Build history of the part. All positions in model axes, mm. A direction names the side the tool comes from. Round coordinates to 2 decimals unless told otherwise and drop trailing zeros. Loops run counter-clockwise (first coordinate to the right, second up) from the corner with the lowest first, then second, coordinate; pieces in that order, holes last. Notation, with made-up numbers: (-7, 70.5) - (40, 70.5) arc R13 cw to (40, 89.5) - close; hole circle Ø9 at (-3, -39). An arc over 180 degrees is marked (long way). Put each result on its own line as item: value. Start each with the question number.
from build123d import *

# Parameters (mm, degrees)
ESQUISSE1_R             = 12.5
BOSS_EXTRU_1_DEPTH      = 54.5
ESQUISSE2_R             = 4
BOSS_EXTRU_2_DEPTH      = 1.35
ESQUISSE3_R             = 1.5
BOSS_EXTRU_3_DEPTH      = 15.7
ESQUISSE4_R             = 13
BOSS_EXTRU_4_DEPTH      = 32.9
ESQUISSE5_R             = 7.5
BOSS_EXTRU_5_DEPTH      = 2
ESQUISSE7_R             = 3
BOSS_EXTRU_6_DEPTH      = 20.8
ESQUISSE8_W             = 9.608231015
ESQUISSE8_H             = 12.440367957
ENL_V_MAT_EXTRU_1_DEPTH = 12
ESQUISSE9_R             = 1.5
ENL_V_MAT_EXTRU_2_DEPTH = 12
ESQUISSE10_R            = 13.05
BOSS_EXTRU_7_DEPTH      = 27
ESQUISSE11_R            = 12.55
BOSS_EXTRU_8_DEPTH      = 3
ESQUISSE12_R            = 1
ENL_V_MAT_EXTRU_4_DEPTH = 1


with BuildPart() as part:
    # Esquisse1 → Boss.-Extru.1 (new body)
    with BuildSketch(Plane.XY):
        Circle(ESQUISSE1_R)
    extrude(amount=BOSS_EXTRU_1_DEPTH)

    # Esquisse2 → Boss.-Extru.2 (add)
    with BuildSketch(Plane(origin=(0, 0, 0), x_dir=(-1, 0, 0), z_dir=(0, 0, -1))):
        with Locations(Location((0, 0, 0), (0, 0, 180))):
            Circle(ESQUISSE2_R)
    extrude(amount=BOSS_EXTRU_2_DEPTH)

    # Esquisse3 → Boss.-Extru.3 (add)
    with BuildSketch(Plane(origin=(0, 0, 0), x_dir=(-1, 0, 0), z_dir=(0, 0, -1))):
        Circle(ESQUISSE3_R)
    extrude(amount=BOSS_EXTRU_3_DEPTH)

    # Esquisse4 → Boss.-Extru.4 (add)
    with BuildSketch(Plane.XY.offset(54.5)):
        Circle(ESQUISSE4_R)
    extrude(amount=BOSS_EXTRU_4_DEPTH)

    # Esquisse5 → Boss.-Extru.5 (add)
    with BuildSketch(Plane.XY.offset(87.4)):
        Circle(ESQUISSE5_R)
    extrude(amount=BOSS_EXTRU_5_DEPTH)

    # Esquisse7 → Boss.-Extru.6 (add)
    with BuildSketch(Plane.XY.offset(87.4)):
        Circle(ESQUISSE7_R)
    extrude(amount=BOSS_EXTRU_6_DEPTH)

    # Esquisse8 → Enlèv. mat.-Extru.1 (cut)
    with BuildSketch(Plane.XY.offset(108.2)):
        with Locations((-0.725995737, 8.720183978)):
            Rectangle(ESQUISSE8_W, ESQUISSE8_H)
    extrude(amount=-ENL_V_MAT_EXTRU_1_DEPTH, mode=Mode.SUBTRACT)

    # Esquisse9 → Enlèv. mat.-Extru.2 (cut)
    with BuildSketch(Plane.XY.offset(87.4)):
        with Locations((-9.999727195, 0)):
            Circle(ESQUISSE9_R)
        with Locations((9.999727195, 0)):
            Circle(ESQUISSE9_R)
        with Locations((0, -10.073864879)):
            Circle(ESQUISSE9_R)
        with Locations((0, 9.926135121)):
            Circle(ESQUISSE9_R)
    extrude(amount=-ENL_V_MAT_EXTRU_2_DEPTH, mode=Mode.SUBTRACT)

    # Esquisse10 → Boss.-Extru.7 (add)
    with BuildSketch(Plane(origin=(0, 0, 54.5), x_dir=(-1, 0, 0), z_dir=(0, 0, -1))):
        Circle(ESQUISSE10_R)
    extrude(amount=-BOSS_EXTRU_7_DEPTH)

    # Esquisse11 → Boss.-Extru.8 (add)
    with BuildSketch(Plane(origin=(0, 0, 0), x_dir=(-1, 0, 0), z_dir=(0, 0, -1))):
        Circle(ESQUISSE11_R)
    extrude(amount=-BOSS_EXTRU_8_DEPTH)

    # Esquisse12 → Enlèv. mat.-Extru.4 (cut)
    with BuildSketch(Plane(origin=(0, 0, 0), x_dir=(-1, 0, 0), z_dir=(0, 0, -1))):
        with Locations((0, 8.5)):
            Circle(ESQUISSE12_R)
        with Locations((7.361215932, -4.25)):
            Circle(ESQUISSE12_R)
        with Locations((0, -8.5)):
            Circle(ESQUISSE12_R)
        with Locations((-7.361215932, -4.25)):
            Circle(ESQUISSE12_R)
        with BuildLine():
            Line((12.364465213, 2.15), (10.005928826, 2.15))
            Line((10.005928826, 2.15), (10.005928826, -0.65))
            Line((10.005928826, -0.65), (12.533156027, -0.65))
            ThreePointArc((12.533156027, -0.65), (12.527285654, 0.754727863), (12.364465213, 2.15))
        make_face()
        with BuildLine():
            Line((-12.533156027, -0.65), (-10.068828371, -0.65))
            Line((-10.068828371, -0.65), (-10.068828371, 2.15))
            Line((-10.068828371, 2.15), (-12.364465213, 2.15))
            ThreePointArc((-12.364465213, 2.15), (-12.527285654, 0.754727863), (-12.533156027, -0.65))
        make_face()
    extrude(amount=-ENL_V_MAT_EXTRU_4_DEPTH, mode=Mode.SUBTRACT)


solid = part.part
1) Drill centre lines: line 1 (Y direction, x = 0, z = 83.15); line 2 (Z direction, x = -1, y = -3.25); line 3 (Z direction, x = -11, y = -5.25). Where is each one in solid material? Low to high. Write a range as [from, to].
2) Pull direction Y, two halves, no side cores. Call faces 5 (the face through (3.2, 0.1, 89.4)), 6 (the face through (8.098, -3.574, 0.493)), 7 (the face through (-11.59, -4.81, 1.48)): pulls with the +Y half, pulls with the -Y half, needs draft (parallel to the pull), parting line crosses it, or undercut.
3) Slice it at B-B, the plane z = 95. Write the cut outline in (x, y), and give its area (3 significant figures).
4) Slice it at A-A, the plane z = 25. Write the cut outline in (x, y), and give its area (3 significant figures).
5) Which spindle directions (+Z, -Z, +X, -X, +Y, -Y) get a long thin tool onto all of the face, cutting with end or side? Do faces 1 (the face through (0, 0, -15.7)), 2 (the face through (-0.65, -2.93, 98.67)), 3 (the face through (1.5, 0.07, -8.42)), 4 (the face through (-11, 1, 1)). Say none if no direction does.
6) Drop flat-ended pins along their axis: pin 1 Ø3 at (x, z) = (-2, 22) entering from -Y; pin 2 Ø3.5 at (x, y) = (0, -10.07) entering from +Z; pin 3 Ø4 at (y, z) = (9.5, 42.5) entering from +X; pin 4 Ø13 at (x, y) = (3.5, 2.5) entering from +Z. Give the stop position or say it passes through.
Taken from the geometry:
1. line 1: y = [-13, -11.57], [-8.57, 8.43], [11.43, 13]
1. line 2: z = [-1.35, 89.4]
1. line 3: z = [0, 87.4]
2. face 5: needs draft
2. face 6: undercut
2. face 7: parting line crosses it
3. outline: circle Ø6 at (0, 0)
3. area: 28.3 mm2
4. outline: circle Ø25 at (0, 0)
4. area: 491 mm2
5. face 1: -Z, +X, -X, +Y, -Y
5. face 2: +Z
5. face 3: -Z
5. face 4: -Z, -X
6. pin 1: stops at y = -12.49
6. pin 2: stops at z = 87.4
6. pin 3: stops at x = 10
6. pin 4: stops at z = 108.2
